The listing builds one solid part. Answer for the finished solid, in the listing's coordinates (mm). A direction names the side the tool comes from. Coordinates: 2 decimals unless noted, no trailing zeros. Write each loop counter-clockwise with the first axis right and the second up, starting at its lowest first coordinate (ties: lowest second). Pieces come first, ordered by that corner, then holes.
Autodesk Inventor part; units mm, degrees
ref_plane "YZ Plane" through (0, 0, 0) normal (1, 0, 0) x (0, 1, 0)
ref_plane "XZ Plane" through (0, 0, 0) normal (0, 1, 0) x (-1, 0, 0)
ref_plane "XY Plane" through (0, 0, 0) normal (0, 0, 1) x (1, 0, 0)
sketch "Sketch1" plane through (0, 0, 0) normal (0, 1, 0) x (-1, 0, 0)
  circle A0 centre (0, 0) radius 25
  circle A1 centre (0, 0) radius 32.5
  dimension "d0" = 50
  dimension "d1" = 65
extrude "Extrusion1" add sketch "Sketch1" along normal blind 7
sketch "Sketch2" plane through (0, 7, 0) normal (0, 1, 0) x (1, 0, 0)
  circle A0 centre (0, 0) radius 27
  circle A1 centre (0, 0) radius 30
  dimension "d4" = 54
  dimension "d5" = 60
extrude "Extrusion2" cut sketch "Sketch2" against normal blind 0.7
sketch "Sketch3" plane through (0, 0, 0) normal (0, -1, 0) x (1, 0, 0)
  circle A0 centre (0, 0) radius 27
  circle A1 centre (0, 0) radius 30
extrude "Extrusion3" cut sketch "Sketch3" against normal blind 0.7
properties part number "bearing_6810zz" material "Stainless Steel, Austenitic"
(1) Find the intervals of material crossed by probe 1 along Z at (x, y) = (0, 0.5); probe 2 along Z at (x, y) = (0, 1.75); probe 3 along X at (y, z) = (0.5, 12), in increasing order.
(2) For a pull along X with two mould halves and no side action, classify faces 1 (the flat face through (-24, 7, -8)), 2 (the cylindrical face through (-31, 3.45, -9.76)), 3 (the cylindrical face through (-29.97, 6.65, -1.32)) as pulls with the +X half, pulls with the -X half, needs draft (parallel to the pull), parting line crosses it, or undercut.
(3) Section D-D, the plane z = 26 is taken. Write down the section's boundary in (x, y).
(4) Each of these flat-tipped pins is pushed along its axis until it touches: pin 1 (1.5 mm diameter, centred on x = 25, z = 2.5, fed in from -Y); pin 2 (2 mm diameter, centred on x = 24, y = 3, fed in from +Z); pin 3 (1 mm diameter, centred on y = 5, z = 12, fed in from +X); pin 4 (4 mm diameter, centred on y = 2, z = 4, fed in from -X). Where does it stop, or does it pass through?
(5) Section B-B, the plane z = 0 is taken. Write down the section's boundary in (x, y).
(6) Section C-C, the plane y = 5.25 is taken. Write down the section's boundary in (x, z).
(7) Section A-A, the plane x = 0 is taken. Write down the section's boundary in (y, z).
(8) Which of the six approach directions +Z, -Z, +X, -X, +Y, -Y give full straight-line access (tool end or side, diameter ignored) to faces 4 (the cylindrical face through (-5.85, 6.65, 26.36)), 5 (the flat face through (-9, 0, -29)), 6 (the cylindrical face through (-5.85, 0.35, -26.36))?
Solution:
1. probe 1: z = -32.5 to -30, -27 to -25, 25 to 27, 30 to 32.5
1. probe 2: z = -32.5 to -25, 25 to 32.5
1. probe 3: x = -30.2 to -27.5, -24.19 to -21.93, 21.93 to 24.19, 27.5 to 30.2
2. face 1: needs draft
2. face 2: parting line crosses it
2. face 3: undercut
3. outline: (-19.5, 0) - (-14.97, 0) - (-14.97, 0.7) - (-7.28, 0.7) - (-7.28, 0) - (7.28, 0) - (7.28, 0.7) - (14.97, 0.7) - (14.97, 0) - (19.5, 0) - (19.5, 7) - (14.97, 7) - (14.97, 6.3) - (7.28, 6.3) - (7.28, 7) - (-7.28, 7) - (-7.28, 6.3) - (-14.97, 6.3) - (-14.97, 7) - (-19.5, 7) - close
4. pin 1: stops at y = 0
4. pin 2: stops at z = 22.96
4. pin 3: stops at x = 30.4
4. pin 4: stops at x = -32.44
5. outline: (-32.5, 0) - (-30, 0) - (-30, 0.7) - (-27, 0.7) - (-27, 0) - (-25, 0) - (-25, 7) - (-27, 7) - (-27, 6.3) - (-30, 6.3) - (-30, 7) - (-32.5, 7) - close; (25, 0) - (27, 0) - (27, 0.7) - (30, 0.7) - (30, 0) - (32.5, 0) - (32.5, 7) - (30, 7) - (30, 6.3) - (27, 6.3) - (27, 7) - (25, 7) - close
6. outline: circle Ø65 at (0, 0); hole circle Ø50 at (0, 0)
7. outline: (0, -32.5) - (7, -32.5) - (7, -30) - (6.3, -30) - (6.3, -27) - (7, -27) - (7, -25) - (0, -25) - (0, -27) - (0.7, -27) - (0.7, -30) - (0, -30) - close; (0, 25) - (7, 25) - (7, 27) - (6.3, 27) - (6.3, 30) - (7, 30) - (7, 32.5) - (0, 32.5) - (0, 30) - (0.7, 30) - (0.7, 27) - (0, 27) - close
8. face 4: +Y
8. face 5: +Z, -Z, +X, -X, -Y
8. face 6: -Y
